Source: CAD feature listing. Evaluate the final solid. Frame: model axes, mm. Give positions to 0.01 mm unless a question says otherwise; leave off trailing zeros. Loops run counter-clockwise (first coordinate to the right, second up) from the corner with the lowest first, then second, coordinate; pieces in that order, holes last. Notation, with made-up numbers: (18.25, 16) - (32.25, 16) arc R27 ccw to (32.25, 43) - close; hole circle Ø1 at (10.5, 49). An arc over 180 degrees is marked (long way). Write each question's results on one line, items separated by ' | '. Start each with the question number.
(1) Contact query for flat-ended pins moving along their axis: pin 1 (4 mm diameter, centred on y = -1.5, z = 57.5, fed in from +X); pin 2 (3 mm diameter, centred on y = -3.5, z = 69, fed in from +X); pin 3 (3.5 mm diameter, centred on x = 0, y = 0, fed in from -Z). Output: stop coordinate, or through.
(2) Cut plane B-B on z = 62. Return the cut outline in (x, y), then the cut area to 3 significant figures.
(3) Cut plane A-A on y = 4. Return the cut outline in (x, z), then the cut area to 3 significant figures.
(4) Material intervals for line 1 along Y through (x, z) = (0, 11); line 2 along Y through (x, z) = (1.5, 67), sorted ascending. Write a range as [from, to].
(5) Cut plane C-C on y = -3.5. Return the cut outline in (x, z).
Autodesk Inventor part; units mm, degrees
ref_plane "YZ Plane" through (0, 0, 0) normal (1, 0, 0) x (0, 1, 0)
ref_plane "XZ Plane" through (0, 0, 0) normal (0, 1, 0) x (-1, 0, 0)
ref_plane "XY Plane" through (0, 0, 0) normal (0, 0, 1) x (1, 0, 0)
sketch "Skizze1" plane through (0, 0, 0) normal (0, 0, 1) x (1, 0, 0)
  line L0 (-7, 0) -> (7, 0)
  line L1 (0, -7) -> (0, 7)
  circle A0 centre (0, 0) radius 5
  dimension "d0" = 10
extrude "Extrusion1" add sketch "Skizze1" along normal blind 100
sketch "Skizze2" plane through (0, 0, 100) normal (0, 0, 1) x (1, 0, 0)
  point P0 (0, 0)
  point P1 (0, 0)
hole "Bohrung1" at (0, 0, 100) direction (0, 0, -1) diameter 4.134 depth 14.2 tip angle 118
sketch "Skizze3" plane through (0, 0, 0) normal (0, 0, -1) x (-1, 0, 0)
  point P0 (0, 0)
  point P1 (-2.4827, -3.6773)
hole "Bohrung2" at (0, 0, 0) direction (0, 0, 1) diameter 4.134 depth 14.2 tip angle 118
properties part number "24_0497_0014"
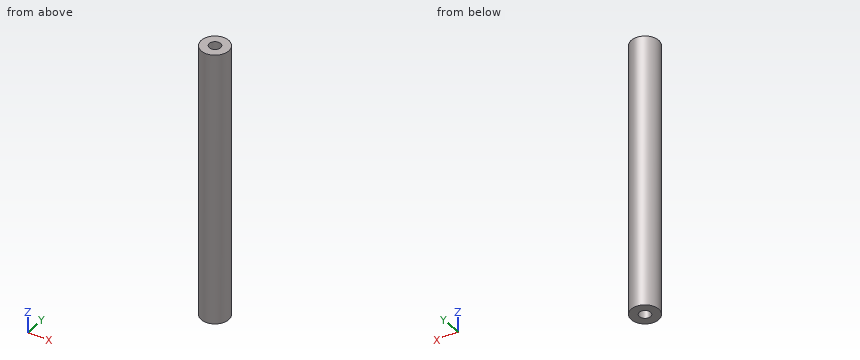
Ans:
1) pin 1: x = 5 | pin 2: x = 4.58 | pin 3: z = 14.39
2) outline: circle Ø10 at (0, 0) | area: 78.5 mm^2
3) outline: (-3, 0) - (3, 0) - (3, 100) - (-3, 100) - close | area: 600 mm^2
4) line 1: [-5, -2.07], [2.07, 5] | line 2: [-4.77, 4.77]
5) outline: (-3.57, 0) - (3.57, 0) - (3.57, 100) - (-3.57, 100) - close
